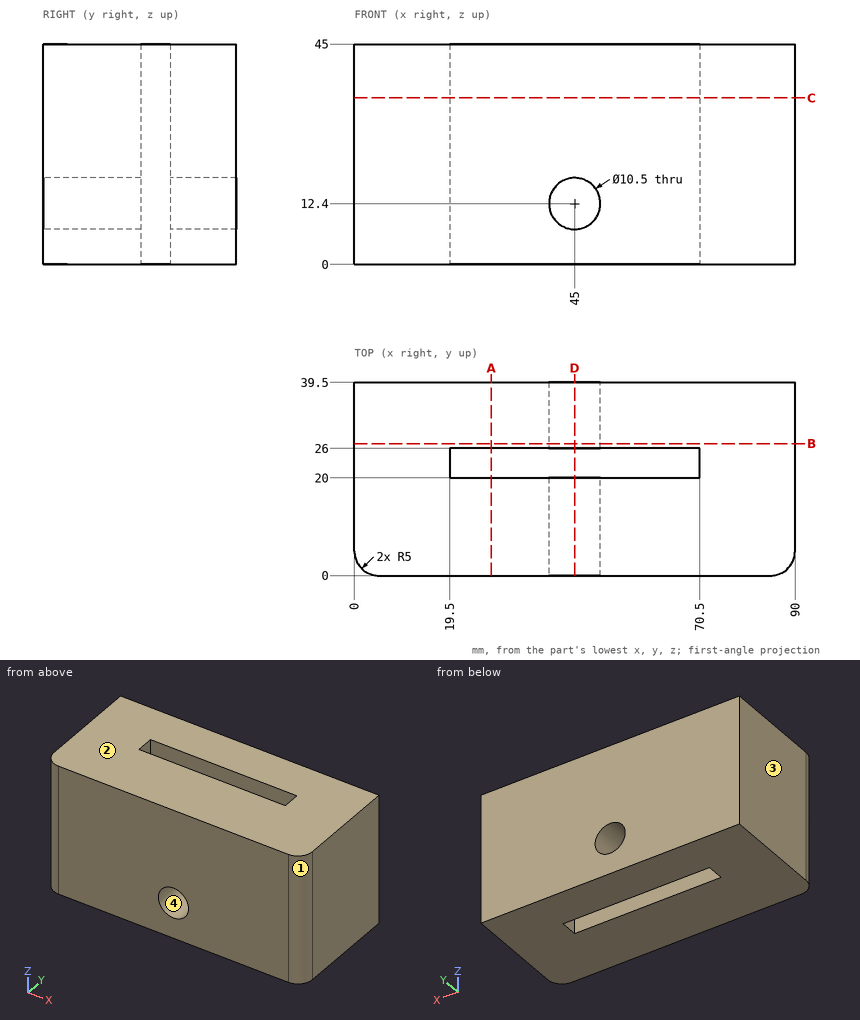
Geometry: see drawing. Coordinates: mm, zero at the bounding-box minimum. Give positions to 0.01 mm unless a question says otherwise; leave off trailing zeros. Write each loop counter-clockwise with the first axis right and the second up, starting at its lowest first coordinate (ties: lowest second). Pieces come first, ordered by that corner, then holes. Notation, with made-up numbers: (33.5, 68) - (78.5, 68) arc R25 cw to (78.5, 88) - close; hole circle Ø6 at (21, 37). An arc over 180 degrees is marked (long way). Return JSON: item names as keys, results as strings. Group by question number.
1) Mould query, pull axis X, two halves, no side actions, for the marked faces 1, 2, 3 and 4. Classes: released by +X, released by -X, zero draft, split by the parting line, or undercut.
2) Section D-D on x = 45. Return the cut outline in (y, z), plus the area to 3 significant figures.
3) Line query: line 1 (Y direction, x = 65, z = 25.5); line 2 (Z direction, x = 45, y = 35); line 3 (X direction, y = 20.5, z = 7). Output: solid intervals per line, ascending.
4) Section C-C on z = 34. Return the cut outline in (x, y), plus the area to 3 significant figures.
5) First-contact query: P1, Ø5, axis at x = 65, z = 11.5, coming from the -Y side; P2, Ø8.5, axis at x = 45, z = 12.4, coming from the +Y side. Flat tips, straight axial feed; report the tip coordinate or a pass-through.
6) Section B-B on y = 27. Return the cut outline in (x, z), plus the area to 3 significant figures.
7) Section A-A on x = 28. Return the cut outline in (y, z).
Filled in:
{
 "1": {"face 1": "released by +X", "face 2": "zero draft", "face 3": "released by -X", "face 4": "undercut"},
 "2": {"outline": "(0, 0) - (20, 0) - (20, 7.15) - (0, 7.15) - close; (0, 17.65) - (20, 17.65) - (20, 45) - (0, 45) - close; (26, 0) - (39.5, 0) - (39.5, 7.15) - (26, 7.15) - close; (26, 17.65) - (39.5, 17.65) - (39.5, 45) - (26, 45) - close", "area": "1,160 mm^2"},
 "3": {"line 1": "y = 0 to 20, 26 to 39.5", "line 2": "z = 0 to 7.15, 17.65 to 45", "line 3": "x = 0 to 19.5, 70.5 to 90"},
 "4": {"outline": "(0, 5) arc R5 ccw to (5, 0) - (85, 0) arc R5 ccw to (90, 5) - (90, 39.5) - (0, 39.5) - close; hole (19.5, 20) - (70.5, 20) - (70.5, 26) - (19.5, 26) - close", "area": "3,240 mm^2"},
 "5": {"P1": "stops at y = 0", "P2": "passes through"},
 "6": {"outline": "(0, 0) - (90, 0) - (90, 45) - (0, 45) - close; hole circle Ø10.5 at (45, 12.4)", "area": "3,960 mm^2"},
 "7": {"outline": "(0, 0) - (20, 0) - (20, 45) - (0, 45) - close; (26, 0) - (39.5, 0) - (39.5, 45) - (26, 45) - close"}
}
